Source: CAD feature listing. Evaluate the final solid. Frame: model axes, mm. Give positions to 0.01 mm unless a question says otherwise; leave off trailing zeros. Order: outer loops, then holes, each group sorted by start corner. A loop starts at its lowest first (then second) coordinate and runs counter-clockwise, first axis right, second up. Notation, with made-up numbers: (83, 45) - (134, 45) arc R24 ccw to (134, 74) - close; hole circle Ø7 at (26, 10.5). An arc over 180 degrees is marked (long way). One line per item, written item: value. Start each with the question number.
from build123d import *

# Parameters (mm, degrees)
F0_W     = 50.8
F0_H     = 129.256198
F1_DEPTH = 25.4
F2_SIZE  = 5.08
F3_R     = 5.868493
F4_DEPTH = 25.4


with BuildPart() as f1:
    # F0 (on Top) → F1 (new body)
    with BuildSketch(Plane.XY):
        with Locations((-31.694914, 4.688799)):
            Rectangle(F0_W, F0_H)
    extrude(amount=-F1_DEPTH)

    # F2
    f2_edges = [f1.edges().sort_by_distance(p)[0] for p in [
        (-57.094914, 4.688799, 0),
        (-31.694914, -59.9393, 0),
        (-31.694914, 69.316898, 0),
    ]]
    chamfer(f2_edges, length=F2_SIZE)

    # F3 (on face) → F4 (cut)
    with BuildSketch(Plane.XY):
        with Locations((-36.104809, 0)):
            Circle(F3_R)
    extrude(amount=-F4_DEPTH, mode=Mode.SUBTRACT)


solid = f1.part
1. Draft query along X for faces 1 (the cylindrical face through (-30.684, -2.248, -12.522)), 2 (the flat face through (-6.295, 4, -13)), 3 (the flat face through (-32.051, 66.741, -2.504)). Return one class per face: pulls with the +X half, pulls with the -X half, needs draft (parallel to the pull), parting line crosses it, or undercut.
2. Section D-D on z = -2. Return the cut outline in (x, y).
3. Section C-C on z = -21.25. Return the cut outline in (x, y).
4. Section B-B on x = -32.5. Return the cut outline in (y, z), then the cut area to 3 significant figures.
5. Section A-A on y = 0. Return the cut outline in (x, z), then the cut area to 3 significant figures.
6. Ray query, L1, parallel to X at y = -1.5, z = -23.75; L2, parallel to Y at x = -37.5, z = -13; L3, parallel to Y at x = -8, z = -4.5. Return the intervals inside material, ascending.
Data:
1. face 1: undercut
1. face 2: pulls with the +X half
1. face 3: needs draft
2. outline: (-54.01, -56.86) - (-6.29, -56.86) - (-6.29, 66.24) - (-54.01, 66.24) - close; hole circle Ø11.74 at (-36.1, 0)
3. outline: (-57.09, -59.94) - (-6.29, -59.94) - (-6.29, 69.32) - (-57.09, 69.32) - close; hole circle Ø11.74 at (-36.1, 0)
4. outline: (-59.94, -25.4) - (-4.63, -25.4) - (-4.63, 0) - (-54.86, 0) - (-59.94, -5.08) - close; (4.63, -25.4) - (69.32, -25.4) - (69.32, -5.08) - (64.24, 0) - (4.63, 0) - close
4. area: 3,020 mm2
5. outline: (-57.09, -25.4) - (-41.97, -25.4) - (-41.97, 0) - (-52.01, 0) - (-57.09, -5.08) - close; (-30.24, -25.4) - (-6.29, -25.4) - (-6.29, 0) - (-30.24, 0) - close
5. area: 979 mm2
6. L1: x = -57.09 to -41.78, -30.43 to -6.29
6. L2: y = -59.94 to -5.7, 5.7 to 69.32
6. L3: y = -59.36 to 68.74
